Source: three-view drawing plus pictorial views. Frame: mm from the lowest corner of the part. A direction names the side the tool comes from. Give positions to 0.01 mm unless a question says otherwise; leave off trailing zeros. Loops run counter-clockwise (first coordinate to the right, second up) from the corner with the lowest first, then second, coordinate; pieces in that order, holes last. Notation, with made-up numbers: M 78,56 L 94,56 A27 cw 94,81 Z; hole C -11.75,77.5 d5. An arc over 180 degrees is marked long. One line per item, written item: value. Start each with the question number.
(1) Access query for the marked faces 5 and 6. Directions: +Z, -Z, +X, -X, +Y, -Y. A direction counts if a zero-diameter tool reaches every point of the face in a straight line with its end or side. Return the directions, or none.
(2) Section B-B on x = 13. Output: boundary loops of the cut face in (y, z).
(3) Pull-direction query (Z, two-part tool) for the marked faces 1, 2, 3 and 4; classes: released by +Z, released by -Z, zero draft, split by the parting line, or undercut.
(4) Section A-A on y = 54. Output: boundary loops of the cut face in (x, z).
(5) Section C-C on y = 30. Output: boundary loops of the cut face in (x, z).
(6) Pin query (flat end, axial travel): P1, Ø1.5, axis at x = 17.5, z = 21, coming from the -Y side; P2, Ø12, axis at y = 48, z = 71, coming from the +X side; P3, Ø1, axis at x = 9, z = 70.5, coming from the +Y side. Return the tip coordinate at first contact, or that it passes through.
(7) Ray query, line 1 along Z through (x, y) = (49, 12.5); line 2 along X through (y, z) = (27.5, 58); line 3 along X through (y, z) = (33, 31). Return the intervals inside material, ascending. Write a range as from..to.
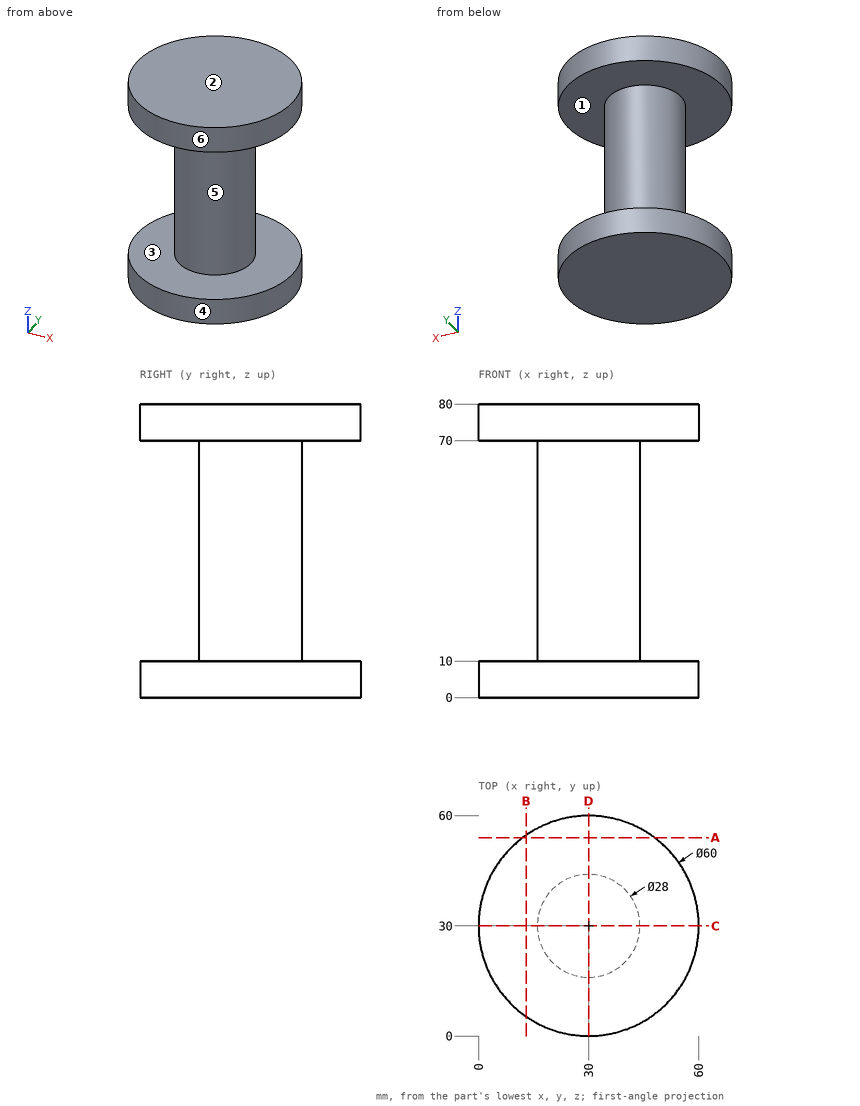
Output values:
1. face 5: none
1. face 6: +Z, -Z
2. outline: M 5.28,0 L 54.72,0 L 54.72,10 L 5.28,10 Z; M 5.28,70 L 54.72,70 L 54.72,80 L 5.28,80 Z
3. face 1: undercut
3. face 2: released by +Z
3. face 3: undercut
3. face 4: zero draft
4. outline: M 12,0 L 48,0 L 48,10 L 12,10 Z; M 12,70 L 48,70 L 48,80 L 12,80 Z
5. outline: M 0,0 L 60,0 L 60,10 L 44,10 L 44,70 L 60,70 L 60,80 L 0,80 L 0,70 L 16,70 L 16,10 L 0,10 Z
6. P1: stops at y = 22.39
6. P2: stops at x = 57.5
6. P3: stops at y = 51.9
7. line 1: z = 0..10, 70..80
7. line 2: x = 16.23..43.77
7. line 3: x = 16.33..43.67
